```python
from build123d import *

# Parameters (mm, degrees)
BOSS_EXTRUDE1_START = 38.1
BOSS_EXTRUDE1_DEPTH = 7.62
FILLET1_R           = 6.35
SKETCH3_R           = 2.54
BOSS_EXTRUDE2_DEPTH = 43.18
SKETCH4_R           = 35.56
BOSS_EXTRUDE3_DEPTH = 60.96


with BuildPart() as part:
    # Sketch1 → Boss-Extrude1 (new body)
    with BuildSketch(Plane(origin=(0, 0, 0), x_dir=(1, 0, 0), z_dir=(0, 1, 0)).offset(BOSS_EXTRUDE1_START)):
        with BuildLine():
            Line((-38.1, -0.419392835), (-23.955144175, -40.544743901))
            ThreePointArc((-23.955144175, -40.544743901), (0, -57.500155839), (23.955144175, -40.544743901))
            Line((23.955144175, -40.544743901), (38.1, -0.419392835))
            Line((38.1, -0.419392835), (38.1, 56.799844161))
            Line((38.1, 56.799844161), (-38.1, 56.799844161))
            Line((-38.1, 56.799844161), (-38.1, -0.419392835))
        make_face()
    extrude(amount=BOSS_EXTRUDE1_DEPTH)

    # Fillet1
    fillet1_edges = [part.edges().sort_by_distance(p)[0] for p in [
        (-38.1, 41.91, -56.799844161),
        (38.1, 41.91, -56.799844161),
    ]]
    fillet(fillet1_edges, radius=FILLET1_R)

    # Sketch3 → Boss-Extrude2 (add)
    with BuildSketch(Plane(origin=(0, 45.72, 0), x_dir=(1, 0, 0), z_dir=(0, 1, 0))):
        with Locations(Location((-31.75, 50.449844161, 0), (0, 0, 270))):
            Circle(SKETCH3_R)
        with Locations(Location((31.75, 50.449844161, 0), (0, 0, 270))):
            Circle(SKETCH3_R)
        with Locations(Location((-14.154646808, -21.090423745, 0), (0, 0, 270))):
            Circle(SKETCH3_R)
        with Locations(Location((14.154646808, -21.090423745, 0), (0, 0, 270))):
            Circle(SKETCH3_R)
    extrude(amount=-BOSS_EXTRUDE2_DEPTH)

    # Sketch4 → Boss-Extrude3 (add)
    with BuildSketch(Plane(origin=(0, 45.72, 0), x_dir=(1, 0, 0), z_dir=(0, 1, 0))):
        with Locations(Location((0, 19.969844161, 0), (0, 0, 90))):
            Circle(SKETCH4_R)
    extrude(amount=BOSS_EXTRUDE3_DEPTH)


solid = part.part
```
Design review of the part built by this model. Coordinates are the model's own, in mm. A direction names the side the tool comes from. Coordinates: 2 decimals unless noted, no trailing zeros. Order: outer loops, then holes, each group sorted by start corner. A loop starts at its lowest first (then second) coordinate and runs counter-clockwise, first axis right, second up. Notation, with made-up numbers: M -17,36.5 L 3,36.5 A27 ccw 3,72.5 Z; hole C 2,54.5 d11. An arc over 180 degrees is marked long. Answer as a JSON object with one key per item and string values. Group by question number.
1) Wall thickness on L1, parallel to X at y = 28.5, z = 21; L2, parallel to Y at x = 6, z = 22; L3, parallel to Y at x = -23.5, z = -46: over which ranges is each line inside the solid? List them lowest first.
2) Mouldability with a two-part tool opening along X and no side actions: class faces 4 (the flat face through (0, 106.68, -19)), 5 (the cylindrical face through (-16.634, 20.569, 20.54)), 6 (the cylindrical face through (-36.19, 41.96, -54.99)), 7 (the cylindrical face through (16.296, 20.569, 22.456)) as pulls with the +X half, pulls with the -X half, needs draft (parallel to the pull), parting line crosses it, or undercut.
3) Add section A-A, the plane x = 0. Write out the cut boundary in (y, z).
4) Add section D-D, the plane y = 59. Write out the cut boundary in (x, z), then the cut area to 3 significant figures.
5) For pin 1 (8 mm diameter, centred on x = 15.5, z = 39.5, fed in from +Y); pin 2 (6 mm diameter, centred on x = 11, z = 32, fed in from -Y); pin 3 (4 mm diameter, centred on y = 92.5, z = -43, fed in from -X), all flat-tipped, find the tip position at first contact; note any pin that passes through.
6) Add section C-C, the plane y = 26. Write out the cut boundary in (x, z), then the cut area to 3 significant figures.
7) Tool access review of faces 1 (the flat face through (-32, 2.54, -50)), 2 (the cylindrical face through (34.714, 75.773, -12.261)), 3 (the cylindrical face through (-30.987, 20.569, -48.027)): name each direction out of +Z, -Z, +X, -X, +Y, -Y from which nothing blocks a thin tool from reaching the whole face with its end or side.
8) Add section B-B, the plane z = -45. Write out the cut boundary in (x, y), then the cut area to 3 significant figures.
Computed values:
{
 "1": {"L1": "x = -16.69 to -11.62, 11.62 to 16.69", "L2": "y = 38.1 to 45.72", "L3": "y = 38.1 to 106.68"},
 "2": {"face 4": "needs draft", "face 5": "undercut", "face 6": "pulls with the -X half", "face 7": "undercut"},
 "3": {"outline": "M 38.1,-56.8 L 45.72,-56.8 L 45.72,-55.53 L 106.68,-55.53 L 106.68,15.59 L 45.72,15.59 L 45.72,57.5 L 38.1,57.5 Z"},
 "4": {"outline": "C 0,-19.97 d71.12", "area": "3,970 mm^2"},
 "5": {"pin 1": "stops at y = 45.72", "pin 2": "stops at y = 38.1", "pin 3": "stops at x = -28.67"},
 "6": {"outline": "C -31.75,-50.45 d5.08; C -14.15,21.09 d5.08; C 14.15,21.09 d5.08; C 31.75,-50.45 d5.08", "area": "81.1 mm^2"},
 "7": {"face 1": "+Z, -Z, +X, -X, -Y", "face 2": "+Y", "face 3": "-Y"},
 "8": {"outline": "M -38.1,38.1 L 38.1,38.1 L 38.1,45.72 L 25.26,45.72 L 25.26,106.68 L -25.26,106.68 L -25.26,45.72 L -38.1,45.72 Z", "area": "3,660 mm^2"}
}
